Read the model definition and answer for the solid it produces. Units are mm, in the model's axes. A direction names the side the tool comes from. Coordinates: 2 decimals unless noted, no trailing zeros. Loops run counter-clockwise (first coordinate to the right, second up) from the corner with the lowest first, then second, coordinate; pieces in that order, holes last. Notation, with made-up numbers: (-16, 3) -> (-12, 3) arc R22 cw to (-12, 35) -> close; hole circle Ø9 at (67, 21). An arc over 180 degrees is marked (long way). Answer in a Markdown table with one row per item.
Autodesk Inventor part; units mm, degrees
ref_plane "YZ Plane" through (0, 0, 0) normal (1, 0, 0) x (0, 1, 0)
ref_plane "XZ Plane" through (0, 0, 0) normal (0, 1, 0) x (-1, 0, 0)
ref_plane "XY Plane" through (0, 0, 0) normal (0, 0, 1) x (1, 0, 0)
sketch "Sketch1" plane through (0, 0, 0) normal (0, 0, 1) x (1, 0, 0)
  line L0 (-12.1708, 16.0073) -> (13.2292, 16.0073)
  line L1 (13.2292, 16.0073) -> (13.2292, -34.7927)
  line L2 (13.2292, -34.7927) -> (-12.1708, -34.7927)
  line L3 (-12.1708, -34.7927) -> (-12.1708, 16.0073)
  line L4 (11.9592, 14.7373) -> (-10.9008, 14.7373)
  line L5 (-10.9008, 14.7373) -> (-10.9008, -33.5227)
  line L6 (-10.9008, -33.5227) -> (11.9592, -33.5227)
  line L7 (11.9592, -33.5227) -> (11.9592, 14.7373)
  point P0 (0, 0)
  dimension "d0" = 25.4
  dimension "d1" = 50.8
  dimension "d2" = 1.27
extrude "Extrusion1" add sketch "Sketch1" along normal blind 660.4
sketch "Sketch2" plane through (-12.1708, 16.0073, 0) normal (0, 1, 0) x (1, 0, 0)
  circle A0 centre (12.7, -12.7) radius 1.7272
  line L0 (25.4, 0) -> (0, 0)
  line L1 (0, 0) -> (0, -660.4)
  point P0 (12.1708, 0)
  dimension "d5" = 3.4544
  dimension "d6" = 12.7
  dimension "d7" = 12.7
extrude "Extrusion2" cut sketch "Sketch2" against normal through all
pattern_linear "Rectangular Pattern1" count 66 spacing 25.4 along (0, 0, 1) of "Extrusion2"
equation "\"d3\" = d13"
equation "\"d10\" = d14"
equation "\"d13\" = 660.4"
equation "\"d14\" = d13"
properties part number "VersaFrame(Towers Top CrossBar)"
1. Given pin 1 Ø4.5 at (x, z) = (0.53, 215.9) entering from -Y, flat-ended and moving along its own axis, determine where the tip first touches the part or whether it passes through.
A:
| item | result |
|---|---|
| pin 1 | stops at y = -34.79 |
2. A tool of negligible diameter and unlimited length cuts with its end or side. For faces 1 (the flat face through (0, -33.523, 326)), 2 (the flat face through (-12.171, -10, 326)), from which of +Z, -Z, +X, -X, +Y, -Y can it reach the whole face along a straight path? Write none if from no direction.
A:
| item | result |
|---|---|
| face 1 | +Z, -Z |
| face 2 | +Z, -Z, -X, +Y, -Y |
3. A cutting plane is placed at B-B on z = 589. Give the vertices of the cut face in (x, y).
A:
| item | result |
|---|---|
| outline | (-12.17, -34.79) -> (13.23, -34.79) -> (13.23, 16.01) -> (-12.17, 16.01) -> close; hole (-10.9, -33.52) -> (11.96, -33.52) -> (11.96, 14.74) -> (-10.9, 14.74) -> close |
4. The mould has two halves that part along X. Classify faces 3 (the flat face through (1, 14.737, 326)), 4 (the flat face through (1, -34.793, 326)), 5 (the flat face through (13.229, -9, 326)): pulls with the +X half, pulls with the -X half, needs draft (parallel to the pull), parting line crosses it, or undercut.
A:
| item | result |
|---|---|
| face 3 | undercut |
| face 4 | needs draft |
| face 5 | pulls with the +X half |
5. Find the intervals of material crossed by probe 1 along X at (y, z) = (-19, 583); probe 2 along Y at (x, z) = (6.5, 413.5); probe 3 along X at (y, z) = (-34, 317), in increasing order.
A:
| item | result |
|---|---|
| probe 1 | x = -12.17 to -10.9, 11.96 to 13.23 |
| probe 2 | y = -34.79 to -33.52, 14.74 to 16.01 |
| probe 3 | x = -12.17 to -1.12, 2.18 to 13.23 |
6. A cutting plane is placed at A-A on y = -4. Give the vertices of the cut face in (x, z), and give its area (3 significant figures).
A:
| item | result |
|---|---|
| outline | (-12.17, 0) -> (-10.9, 0) -> (-10.9, 660.4) -> (-12.17, 660.4) -> close; (11.96, 0) -> (13.23, 0) -> (13.23, 660.4) -> (11.96, 660.4) -> close |
| area | 1,680 mm2 |
